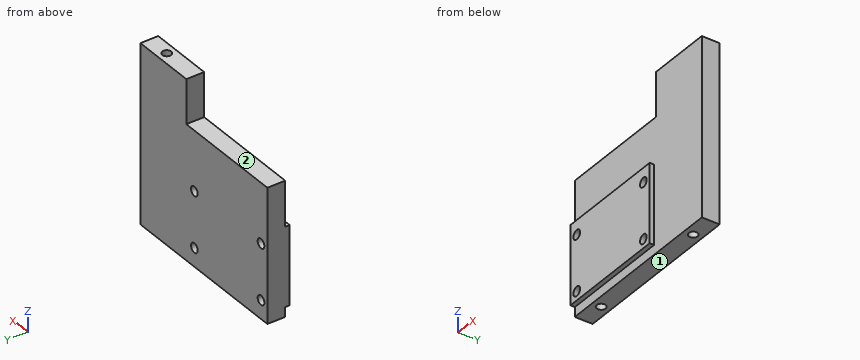
from build123d import *

# Parameters (mm, degrees)
SKETCH1_W           = 40
SKETCH1_H           = 40
BOSS_EXTRUDE1_DEPTH = 4
SKETCH4_R           = 1
CUT_EXTRUDE2_DEPTH  = 2
SKETCH5_R           = 1
CUT_EXTRUDE3_DEPTH  = 2
SKETCH6_W           = 25
SKETCH6_H           = 17.723883745
SKETCH6_R           = 1.05
BOSS_EXTRUDE3_DEPTH = 1
SKETCH8_R           = 1.05
CUT_EXTRUDE4_DEPTH  = 29.722813233
SKETCH9_W           = 25.523793116
SKETCH9_H           = 9.941729438
CUT_EXTRUDE5_DEPTH  = 29.565713714


with BuildPart() as part:
    # Sketch1 → Boss-Extrude1 (new body)
    with BuildSketch(Plane(origin=(0, 0, 0), x_dir=(1, 0, 0), z_dir=(0, 1, 0))):
        Rectangle(SKETCH1_W, SKETCH1_H)
    extrude(amount=BOSS_EXTRUDE1_DEPTH)

    # Sketch4 → Cut-Extrude2 (cut)
    with BuildSketch(Plane.XY.offset(20)):
        with Locations((-14.5, 2)):
            Circle(SKETCH4_R)
        with Locations((14.5, 2)):
            Circle(SKETCH4_R)
    extrude(amount=-CUT_EXTRUDE2_DEPTH, mode=Mode.SUBTRACT)

    # Sketch5 → Cut-Extrude3 (cut)
    with BuildSketch(Plane(origin=(0, 0, -20), x_dir=(-1, 0, 0), z_dir=(0, 0, -1))):
        with Locations(Location((-14.5, 2, 0), (0, 0, 180))):
            Circle(SKETCH5_R)
        with Locations(Location((14.5, 2, 0), (0, 0, 180))):
            Circle(SKETCH5_R)
    extrude(amount=-CUT_EXTRUDE3_DEPTH, mode=Mode.SUBTRACT)

    # Sketch6 → Boss-Extrude3 (add)
    with BuildSketch(Plane(origin=(0, 0, 0), x_dir=(-1, 0, 0), z_dir=(0, -1, 0))):
        with Locations((7.5, 8.985238628)):
            Rectangle(SKETCH6_W, SKETCH6_H)
        with Locations(Location((17.998887809, 15.84606831, 0), (0, 0, 90))):
            Circle(SKETCH6_R, mode=Mode.SUBTRACT)
        with Locations(Location((-2.998887809, 15.84606831, 0), (0, 0, 90))):
            Circle(SKETCH6_R, mode=Mode.SUBTRACT)
        with Locations(Location((-2.998887809, 3.34606831, 0), (0, 0, 90))):
            Circle(SKETCH6_R, mode=Mode.SUBTRACT)
        with Locations(Location((17.998887809, 3.34606831, 0), (0, 0, 90))):
            Circle(SKETCH6_R, mode=Mode.SUBTRACT)
    extrude(amount=BOSS_EXTRUDE3_DEPTH)

    # Sketch8 → Cut-Extrude4 (cut, through all)
    with BuildSketch(Plane.XZ.offset(1)):
        with Locations(Location((-17.998887809, -15.84606831, 0), (0, 0, 270))):
            Circle(SKETCH8_R)
        with Locations(Location((2.998887809, -15.84606831, 0), (0, 0, 270))):
            Circle(SKETCH8_R)
        with Locations(Location((2.998887809, -3.34606831, 0), (0, 0, 270))):
            Circle(SKETCH8_R)
        with Locations(Location((-17.998887809, -3.34606831, 0), (0, 0, 270))):
            Circle(SKETCH8_R)
    extrude(amount=-CUT_EXTRUDE4_DEPTH, mode=Mode.SUBTRACT)

    # Sketch9 → Cut-Extrude5 (cut, through all)
    with BuildSketch(Plane(origin=(0, 0, 0), x_dir=(-1, 0, 0), z_dir=(0, -1, 0))):
        with Locations((7.238103442, -15.029135281)):
            Rectangle(SKETCH9_W, SKETCH9_H)
    extrude(amount=-CUT_EXTRUDE5_DEPTH, mode=Mode.SUBTRACT)


solid = part.part
Could you check a few things on this model? Use its own coordinates, in mm. Face numbers are marked on the shaded views. A direction names the side the tool comes from. Coordinates: 2 decimals unless noted, no trailing zeros. Write each loop counter-clockwise with the first axis right and the second up, starting at its lowest first coordinate (ties: lowest second). Pieces come first, ordered by that corner, then holes. Notation, with made-up numbers: M 9,69.25 L 31,69.25 A37 cw 31,105.25 Z; hole C 43.5,55 d9. An arc over 180 degrees is marked long. One line per question, with ' | ' between items.
1) For pin 1 Ø0.5 at (x, y) = (-4, -0.5) entering from +Z; pin 2 Ø2.5 at (x, y) = (14.5, 2) entering from -Z; pin 3 Ø1.7 at (x, z) = (-18, -3.35) entering from -Y; pin 4 Ø3 at (x, y) = (-14.5, 2) entering from +Z, each with a flat end and sliding along its axis, tell me the tip position at first contact or that it passes through.
Checks:
pin 1: z = -0.12 | pin 2: z = -20 | pin 3: through | pin 4: z = 10.06
2) I need wall thicknesses on probe 1 along X at (y, z) = (2, -18.6); probe 2 along X at (y, z) = (1.65, -3); probe 3 along X at (y, z) = (-0.4, -13). Which ranges of each line are inside material? Lowest first, please. Write a range as [from, to].
Checks:
probe 1: [-20, -15.5], [-13.5, 13.5], [15.5, 20] | probe 2: [-20, -18.99], [-17.01, 2.01], [3.99, 20] | probe 3: [-20, 5]
3) Imagine slicing it at B-B, the plane y = 2. Write out the boundary of the cut face in (x, z).
Checks:
outline: M -20,-20 L -15.5,-20 L -15.5,-18 L -13.5,-18 L -13.5,-20 L 13.5,-20 L 13.5,-18 L 15.5,-18 L 15.5,-20 L 20,-20 L 20,20 L 15.5,20 L 15.5,18 L 13.5,18 L 13.5,20 L 5.52,20 L 5.52,10.06 L -20,10.06 Z; hole C -18,-15.85 d2.1; hole C -18,-3.35 d2.1; hole C 3,-15.85 d2.1; hole C 3,-3.35 d2.1
4) Imagine slicing it at D-D, the plane x = 14.5. Write out the boundary of the cut face in (y, z).
Checks:
outline: M 0,-20 L 1,-20 L 1,-18 L 3,-18 L 3,-20 L 4,-20 L 4,20 L 3,20 L 3,18 L 1,18 L 1,20 L 0,20 Z
5) Imagine slicing it at A-A, the plane x = -14.5. Write out the boundary of the cut face in (y, z), and give its area (3 significant figures).
Checks:
outline: M -1,-17.85 L 0,-17.85 L 0,-20 L 1,-20 L 1,-18 L 3,-18 L 3,-20 L 4,-20 L 4,10.06 L 0,10.06 L 0,-0.12 L -1,-0.12 Z | area: 134 mm²
6) For the marked faces 1 and 2, which set-ups out of +Z, -Z, +X, -X, +Y, -Y let a thin tool reach every point of the face, with its end or its side?
Checks:
face 1: -Z, +X, -X, +Y, -Y | face 2: +Z, -X, +Y, -Y
7) Imagine slicing it at C-C, the plane z = -8. Write out the boundary of the cut face in (x, y).
Checks:
outline: M -20,-1 L 5,-1 L 5,0 L 20,0 L 20,4 L -20,4 Z
